Check sheet for the drawn part. Datum: minimum x, y, z corner. Units: mm. A direction names the side the tool comes from. Give positions to 0.01 mm unless a question says otherwise; leave off trailing zeros. Loops run counter-clockwise (first coordinate to the right, second up) from the corner with the lowest first, then second, coordinate; pieces in that order, holes last. Notation, with made-up numbers: (34.25, 47.5) - (86.25, 47.5) arc R5 cw to (86.25, 52.5) - close; hole circle Ø1 at (36, 53). An arc over 180 degrees is marked (long way). Use a Markdown table: item, result. Add a question column.
1. Cross-section at C-C on z = 66.5. Enter the section's corners in (x, y) (1 decimal).
2. Depth check by flat-ended pin: P1, Ø5, axis at y = 19, z = 62.5, coming from the +X side; P2, Ø1, axis at x = 179.5, y = 20, coming from the +Z side; P3, Ø2, axis at y = 12.5, z = 12.5, coming from the -X side; P4, Ø3, axis at y = 17, z = 31, coming from the +X side (1 decimal). Enter the tip coordinate at first touch or a pass-through.
3. Cross-section at B-B on x = 201.5. Enter the section's corners in (y, z), and give its area (3 significant figures).
4. Set-up check for the marked faces 1 and 2: record each of +Z, -Z, +X, -X, +Y, -Y from which the full face is reachable in a straight line by a thin tool's end or side.
5. Material ranges on L1, parallel to Z at x = 70.5, y = 6.5; L2, parallel to Z at x = 212.5, y = 24.25; L3, parallel to X at y = 4.25, z = 61 (1 decimal), recorded low to high.
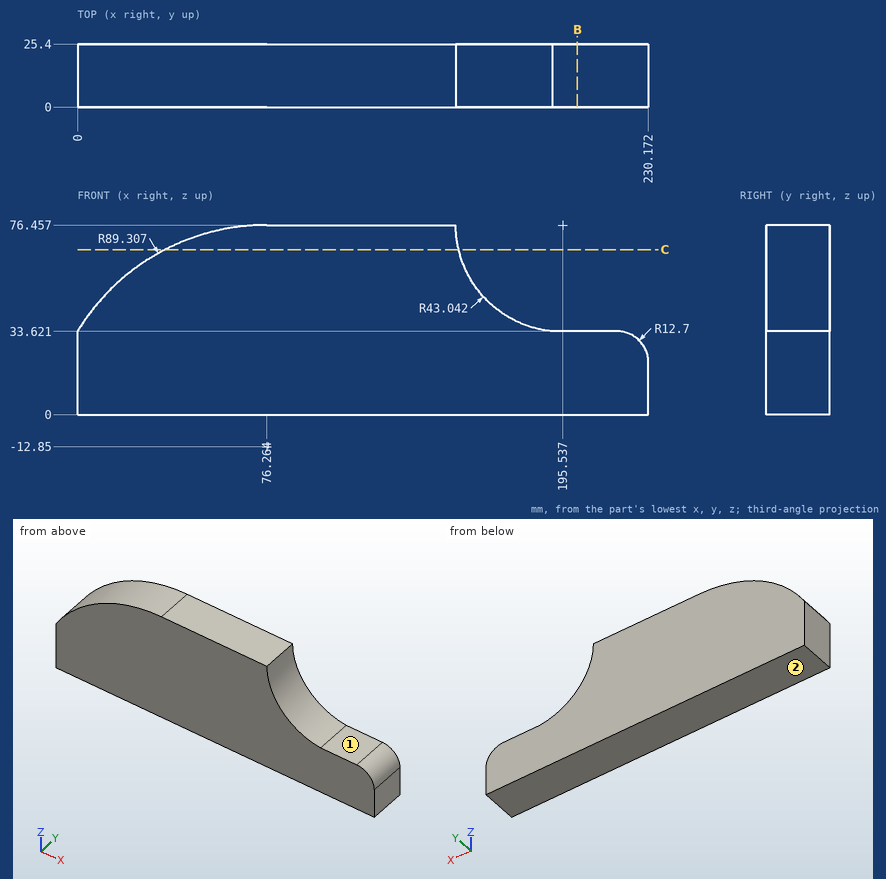
Values found:
| question | item | result |
|---|---|---|
| 1 | outline | (35.3, 0) - (153.7, 0) - (153.7, 25.4) - (35.3, 25.4) - close |
| 2 | P1 | stops at x = 155.77 |
| 2 | P2 | stops at z = 36.72 |
| 2 | P3 | stops at x = 0 |
| 2 | P4 | stops at x = 226.8 |
| 3 | outline | (0, 0) - (25.4, 0) - (25.4, 33.62) - (0, 33.62) - close |
| 3 | area | 854 mm2 |
| 4 | face 1 | +Z, +X, +Y, -Y |
| 4 | face 2 | -Z, +X, -X, +Y, -Y |
| 5 | L1 | z = 0 to 76.27 |
| 5 | L2 | z = 0 to 33.62 |
| 5 | L3 | x = 26 to 155.4 |
